Print and shaded views of the part. All mm, measured from the part's lowest x, y and z. A direction names the side the tool comes from. Coordinates: 2 decimals unless noted, no trailing zeros. Loops run counter-clockwise (first coordinate to the right, second up) from the corner with the lowest first, then second, coordinate; pieces in that order, holes last.
1) Which spindle directions (+Z, -Z, +X, -X, +Y, -Y) get a long thin tool onto all of the face, cutting with end or side? Do the marked faces 4, 5 and 6. Say none if no direction does.
2) Wall check: line 1 along Z through (x, y) = (18.5, 82); line 2 along X through (y, z) = (86, 31.5); line 3 along X through (y, z) = (93, 14.5). Give the ranges that are in metal, low to high.
3) Saw through at D-D, the plane z = 18.5. Write the cut outline in (x, y).
4) Saw through at C-C, the plane y = 84.5. Write the cut outline in (x, z), and give its area (3 significant figures).
5) Saw through at B-B, the plane x = 28. Write the cut outline in (y, z), and give its area (3 significant figures).
6) Two-plate mould, pull along Y, no slides. Class the marked faces 1, 2 and 3: +Y half, -Y half, draft (parallel to the pull), parting line (faces both ways), or undercut.
7) Saw through at A-A, the plane y = 28.5. Write the cut outline in (x, z), and give its area (3 significant figures).
8) Pin check, flat tips, straight feed: pin 1 Ø2 at (x, z) = (38.5, 30) entering from -Y; pin 2 Ø1 at (y, z) = (67, 35.5) entering from -X; pin 3 Ø2.5 at (x, z) = (38.5, 10) entering from -Y. Stop position of each tip, or through.
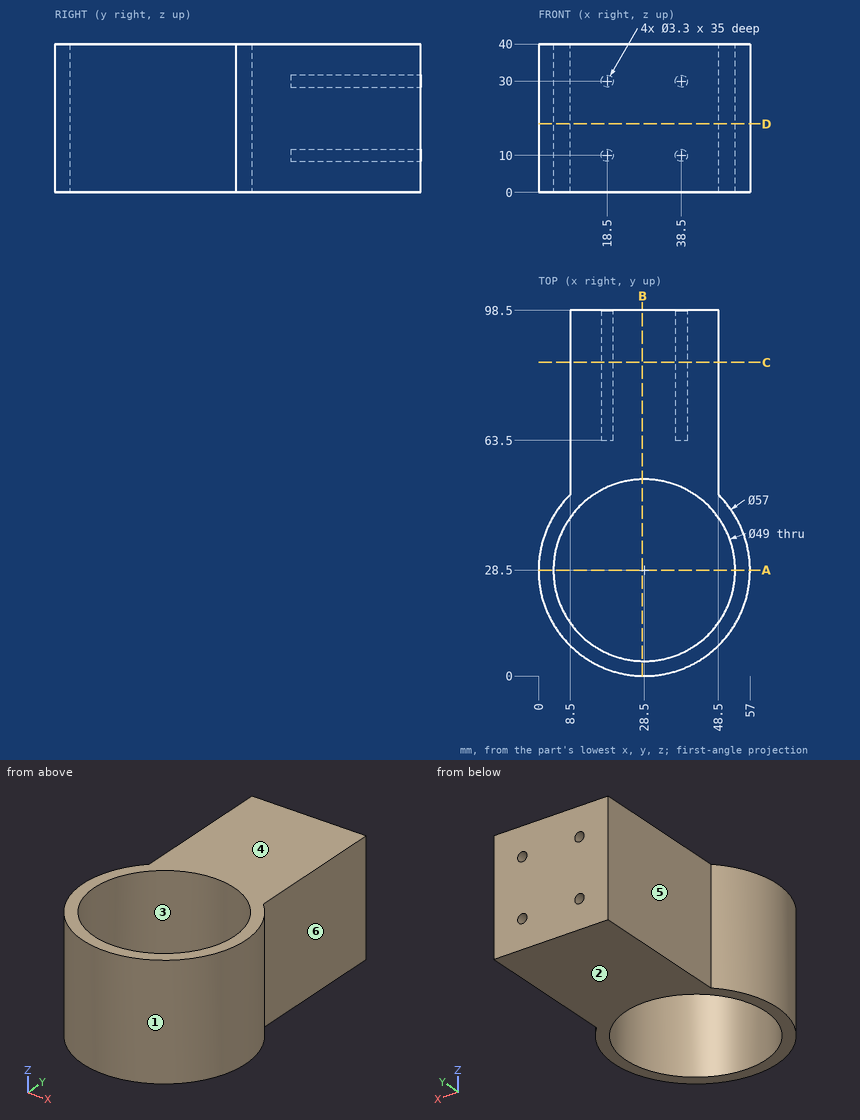
Data:
1. face 4: +Z, +X, -X, +Y, -Y
1. face 5: +Z, -Z, -X, +Y
1. face 6: +Z, -Z, +X, +Y
2. line 1: z = 0 to 8.35, 11.65 to 28.35, 31.65 to 40
2. line 2: x = 8.5 to 17.81, 19.19 to 37.81, 39.19 to 48.5
2. line 3: x = 8.5 to 48.5
3. outline: (8.5, 48.8) arc R28.5 ccw (long way) to (48.5, 48.8) - (48.5, 98.5) - (8.5, 98.5) - close; hole circle Ø49 at (28.5, 28.5)
4. outline: (8.5, 0) - (48.5, 0) - (48.5, 40) - (8.5, 40) - close; hole circle Ø3.3 at (18.5, 10); hole circle Ø3.3 at (18.5, 30); hole circle Ø3.3 at (38.5, 10); hole circle Ø3.3 at (38.5, 30)
4. area: 1,570 mm2
5. outline: (0, 0) - (4.01, 0) - (4.01, 40) - (0, 40) - close; (52.99, 0) - (98.5, 0) - (98.5, 40) - (52.99, 40) - close
5. area: 1,980 mm2
6. face 1: parting line
6. face 2: draft
6. face 3: undercut
7. outline: (0, 0) - (4, 0) - (4, 40) - (0, 40) - close; (53, 0) - (57, 0) - (57, 40) - (53, 40) - close
7. area: 320 mm2
8. pin 1: stops at y = 1.46
8. pin 2: stops at x = 8.5
8. pin 3: stops at y = 1.38
